from build123d import *

# Parameters (mm, degrees)
SALIENTE_EXTRUIR1_DEPTH = 3
CORTAR_EXTRUIR1_REACH   = 5
CROQUIS2_W              = 5
CROQUIS2_H              = 8
CROQUIS3_W              = 10
CROQUIS3_H              = 8
SALIENTE_EXTRUIR2_DEPTH = 35
CORTAR_EXTRUIR2_DEPTH   = 12
REDONDEO1_R             = 2
REDONDEO2_R             = 2
SALIENTE_EXTRUIR3_DEPTH = 59
CORTAR_EXTRUIR3_REACH   = 38.4
CROQUIS6_R              = 1.25
CORTAR_EXTRUIR4_REACH   = 5
CROQUIS7_R              = 1.75
CROQUIS7_W              = 8
CROQUIS7_H              = 20


with BuildPart() as part:
    # Croquis1 → Saliente-Extruir1 (new body)
    with BuildSketch(Plane(origin=(0, 0, 0), x_dir=(1, 0, 0), z_dir=(0, 1, 0))):
        with BuildLine():
            Line((7, 0), (47, 0))
            ThreePointArc((47, 0), (51.949747468, 2.050252532), (54, 7))
            Line((54, 7), (54, 37))
            ThreePointArc((54, 37), (51.949747468, 41.949747468), (47, 44))
            Line((47, 44), (7, 44))
            ThreePointArc((7, 44), (2.050252532, 41.949747468), (0, 37))
            Line((0, 37), (0, 7))
            ThreePointArc((0, 7), (2.050252532, 2.050252532), (7, 0))
        make_face()
    extrude(amount=SALIENTE_EXTRUIR1_DEPTH)

    # Croquis2 → Cortar-Extruir1 (cut, up to next)
    with BuildSketch(Plane(origin=(0, 3, 0), x_dir=(1, 0, 0), z_dir=(0, 1, 0)), mode=Mode.PRIVATE) as cortar_extruir1_sk1:
        with Locations((38.9, 24.5)):
            Rectangle(CROQUIS2_W, CROQUIS2_H)
    cortar_extruir1_tool1 = extrude(cortar_extruir1_sk1.sketch, amount=-CORTAR_EXTRUIR1_REACH, mode=Mode.PRIVATE) & part.part
    add(cortar_extruir1_tool1.solids().sort_by_distance((38.9, 3, -24.5))[0], mode=Mode.SUBTRACT)

    # Croquis3 → Saliente-Extruir2 (add)
    with BuildSketch(Plane(origin=(0, 3, 0), x_dir=(1, 0, 0), z_dir=(0, 1, 0))):
        with Locations((17, 38)):
            Rectangle(CROQUIS3_W, CROQUIS3_H)
        with Locations((17, 6)):
            Rectangle(CROQUIS3_W, CROQUIS3_H)
    extrude(amount=SALIENTE_EXTRUIR2_DEPTH)

    # Croquis4 → Cortar-Extruir2 (cut)
    with BuildSketch(Plane(origin=(0, 38, 0), x_dir=(1, 0, 0), z_dir=(0, 1, 0))):
        with BuildLine():
            Line((14.9, 10.594122727), (14.9, 3.9))
            Line((14.9, 3.9), (16.9, 3.9))
            Line((16.9, 3.9), (16.9, 10.101282262))
            ThreePointArc((16.9, 10.101282262), (15.866874644, 10.213276209), (14.9, 10.594122727))
        make_face()
        with BuildLine():
            Line((16.9, 17.898717738), (16.9, 40.1))
            Line((16.9, 40.1), (14.9, 40.1))
            Line((14.9, 40.1), (14.9, 17.405877273))
            ThreePointArc((14.9, 17.405877273), (15.866874644, 17.786723791), (16.9, 17.898717738))
        make_face()
    extrude(amount=-CORTAR_EXTRUIR2_DEPTH, mode=Mode.SUBTRACT)

    # Redondeo1
    redondeo1_edges = [part.edges().sort_by_distance(p)[0] for p in [
        (12, 20.5, -42),
        (12, 20.5, -2),
    ]]
    fillet(redondeo1_edges, radius=REDONDEO1_R)

    # Redondeo2
    redondeo2_edges = [part.edges().sort_by_distance(p)[0] for p in [
        (17, 3, -34),
        (22, 3, -38),
        (22, 3, -6),
        (17, 3, -10),
    ]]
    fillet(redondeo2_edges, radius=REDONDEO2_R)

    # Croquis5 → Saliente-Extruir3 (add)
    with BuildSketch(Plane(origin=(0, 3, 0), x_dir=(1, 0, 0), z_dir=(0, 1, 0))):
        Polygon((36.4, 34.5), (36.4, 14.5), (24.4, 14.5), (24.4, 34.5), (26.8, 34.5), (26.8, 16.9), (34, 16.9), (34, 34.5), align=None)
    extrude(amount=SALIENTE_EXTRUIR3_DEPTH)

    # Croquis6 → Cortar-Extruir3 (cut, up to next)
    with BuildSketch(Plane(origin=(36.4, 0, 0), x_dir=(0, 0, -1), z_dir=(1, 0, 0)), mode=Mode.PRIVATE) as cortar_extruir3_sk1:
        with Locations((27.4, 47.5)):
            Circle(CROQUIS6_R)
    cortar_extruir3_tool1 = extrude(cortar_extruir3_sk1.sketch, amount=-CORTAR_EXTRUIR3_REACH, mode=Mode.PRIVATE) & part.part
    add(cortar_extruir3_tool1.solids().sort_by_distance((36.4, 47.5, -27.4))[0], mode=Mode.SUBTRACT)
    # Croquis6 → Cortar-Extruir3 (cut, up to next)
    with BuildSketch(Plane(origin=(36.4, 0, 0), x_dir=(0, 0, -1), z_dir=(1, 0, 0)), mode=Mode.PRIVATE) as cortar_extruir3_sk2:
        with Locations((27.4, 19.7)):
            Circle(CROQUIS6_R)
    cortar_extruir3_tool2 = extrude(cortar_extruir3_sk2.sketch, amount=-CORTAR_EXTRUIR3_REACH, mode=Mode.PRIVATE) & part.part
    add(cortar_extruir3_tool2.solids().sort_by_distance((36.4, 19.7, -27.4))[0], mode=Mode.SUBTRACT)

    # Croquis7 → Cortar-Extruir4 (cut, up to next)
    with BuildSketch(Plane(origin=(0, 3, 0), x_dir=(1, 0, 0), z_dir=(0, 1, 0)), mode=Mode.PRIVATE) as cortar_extruir4_sk1:
        with Locations((4, 22)):
            Circle(CROQUIS7_R)
    cortar_extruir4_tool1 = extrude(cortar_extruir4_sk1.sketch, amount=-CORTAR_EXTRUIR4_REACH, mode=Mode.PRIVATE) & part.part
    add(cortar_extruir4_tool1.solids().sort_by_distance((4, 3, -22))[0], mode=Mode.SUBTRACT)
    # Croquis7 → Cortar-Extruir4 (cut, up to next)
    with BuildSketch(Plane(origin=(0, 3, 0), x_dir=(1, 0, 0), z_dir=(0, 1, 0)), mode=Mode.PRIVATE) as cortar_extruir4_sk2:
        with Locations((47, 37)):
            Circle(CROQUIS7_R)
    cortar_extruir4_tool2 = extrude(cortar_extruir4_sk2.sketch, amount=-CORTAR_EXTRUIR4_REACH, mode=Mode.PRIVATE) & part.part
    add(cortar_extruir4_tool2.solids().sort_by_distance((47, 3, -37))[0], mode=Mode.SUBTRACT)
    # Croquis7 → Cortar-Extruir4 (cut, up to next)
    with BuildSketch(Plane(origin=(0, 3, 0), x_dir=(1, 0, 0), z_dir=(0, 1, 0)), mode=Mode.PRIVATE) as cortar_extruir4_sk3:
        with Locations((47, 7)):
            Circle(CROQUIS7_R)
    cortar_extruir4_tool3 = extrude(cortar_extruir4_sk3.sketch, amount=-CORTAR_EXTRUIR4_REACH, mode=Mode.PRIVATE) & part.part
    add(cortar_extruir4_tool3.solids().sort_by_distance((47, 3, -7))[0], mode=Mode.SUBTRACT)
    # Croquis7 → Cortar-Extruir4 (cut, up to next)
    with BuildSketch(Plane(origin=(0, 3, 0), x_dir=(1, 0, 0), z_dir=(0, 1, 0)), mode=Mode.PRIVATE) as cortar_extruir4_sk4:
        with Locations((20, 22)):
            Rectangle(CROQUIS7_W, CROQUIS7_H)
    cortar_extruir4_tool4 = extrude(cortar_extruir4_sk4.sketch, amount=-CORTAR_EXTRUIR4_REACH, mode=Mode.PRIVATE) & part.part
    add(cortar_extruir4_tool4.solids().sort_by_distance((20, 3, -22))[0], mode=Mode.SUBTRACT)


solid = part.part
Geometry: final body of the model. Coordinates: model frame, mm. A direction names the side the tool comes from. Give positions to 0.01 mm unless a question says otherwise; leave off trailing zeros. Write each loop counter-clockwise with the first axis right and the second up, starting at its lowest first coordinate (ties: lowest second). Pieces come first, ordered by that corner, then holes.
(1) Ray query, line 1 (Y direction, x = 34.8, z = -27.4); line 2 (X direction, y = 1, z = -22); line 3 (X direction, y = 6.5, z = -23). Return the intervals inside material, ascending.
(2) Cut plane D-D, the plane z = -30.5. Return loops of the section in (x, y).
(3) Cut plane C-C, the plane y = 8. Return loops of the section in (x, z), then the cut area to 3 significant figures.
(4) Access query for faces 4 (the cylindrical face through (12.6, 20.74, -41.43)), 5 (the flat face through (16, 26, -7)), 6 (the flat face through (39, 2, -28.5)), 7 (the cylindrical face through (35.217, 20.754, -28.072)), 8 (the flat face through (26, 32, -34.5)). Directions: +Z, -Z, +X, -X, +Y, -Y. A direction counts if a zero-diameter tool reaches every point of the face in a straight line with its end or side. Return the directions, or none.
(5) Mould query, pull axis Z, two halves, no side actions, for faces 1 (the flat face through (14.9, 32, -37)), 2 (the flat face through (34.5, 62, -24.6)), 3 (the flat face through (30, 32, -14.5)). Classes: released by +Z, released by -Z, zero draft, split by the parting line, or undercut.
(6) Cut plane A-A, the plane z = -24.5. Return loops of the section in (x, y), then the cut area to 3 significant figures.
(7) Cut plane B-B, the plane y = 47.5. Return loops of the section in (x, z), then the cut area to 3 significant figures.
(8) First-contact query: P1, Ø12, axis at x = 8, z = -37.5, coming from the +Y side; P2, Ø5, axis at y = 29, z = -7.5, coming from the -X side; P3, Ø3.5, axis at x = 31, y = 35, coming from the -Z side. Flat tips, straight axial feed; report the tip coordinate or a pass-through.
Values follow:
1. line 1: y = 0 to 18.45, 20.95 to 46.25, 48.75 to 62
1. line 2: x = 0 to 2.25, 5.75 to 16, 24 to 36.4, 41.4 to 54
1. line 3: x = 24.4 to 26.8, 34 to 36.4
2. outline: (0, 0) - (16, 0) - (16, 3) - (0, 3) - close; (24, 0) - (54, 0) - (54, 3) - (36.4, 3) - (36.4, 62) - (34, 62) - (34, 3) - (26.8, 3) - (26.8, 62) - (24.4, 62) - (24.4, 3) - (24, 3) - close
3. outline: (12, -40) arc R2 ccw to (14, -42) - (22, -42) - (22, -34) - (12, -34) - close; (12, -10) - (22, -10) - (22, -2) - (14, -2) arc R2 ccw to (12, -4) - close; (24.4, -34.5) - (26.8, -34.5) - (26.8, -16.9) - (34, -16.9) - (34, -34.5) - (36.4, -34.5) - (36.4, -14.5) - (24.4, -14.5) - close
3. area: 272 mm2
4. face 4: -Z, -X, +Y
4. face 5: +Y
4. face 6: +Y, -Y
4. face 7: +X
4. face 8: -Z, +X, +Y
5. face 1: undercut
5. face 2: zero draft
5. face 3: released by +Z
6. outline: (0, 0) - (16, 0) - (16, 3) - (0, 3) - close; (24, 0) - (36.4, 0) - (36.4, 62) - (34, 62) - (34, 3) - (26.8, 3) - (26.8, 62) - (24.4, 62) - (24.4, 3) - (24, 3) - close; (41.4, 0) - (54, 0) - (54, 3) - (41.4, 3) - close
6. area: 406 mm2
7. outline: (24.4, -34.5) - (26.8, -34.5) - (26.8, -16.9) - (34, -16.9) - (34, -26.15) - (36.4, -26.15) - (36.4, -14.5) - (24.4, -14.5) - close; (34, -34.5) - (36.4, -34.5) - (36.4, -28.65) - (34, -28.65) - close
7. area: 107 mm2
8. P1: stops at y = 38
8. P2: stops at x = 12
8. P3: stops at z = -16.9
